For this review, use the dimensioned drawing (mm, ordinates from the lowest corner) and the shaded views. A direction names the side the tool comes from. Round coordinates to 2 decimals unless told otherwise and drop trailing zeros. Order: outer loops, then holes, each group sorted by start corner. A loop starts at its lowest first (then second) coordinate and runs counter-clockwise, first axis right, second up. Notation, with made-up numbers: (-31.5, 55) -> (-15.5, 55) arc R23 ccw to (-15.5, 86) -> close; hole circle Ø4 at (78, 72.25). An arc over 180 degrees is marked (long way). Answer in a Markdown table with one row per item.
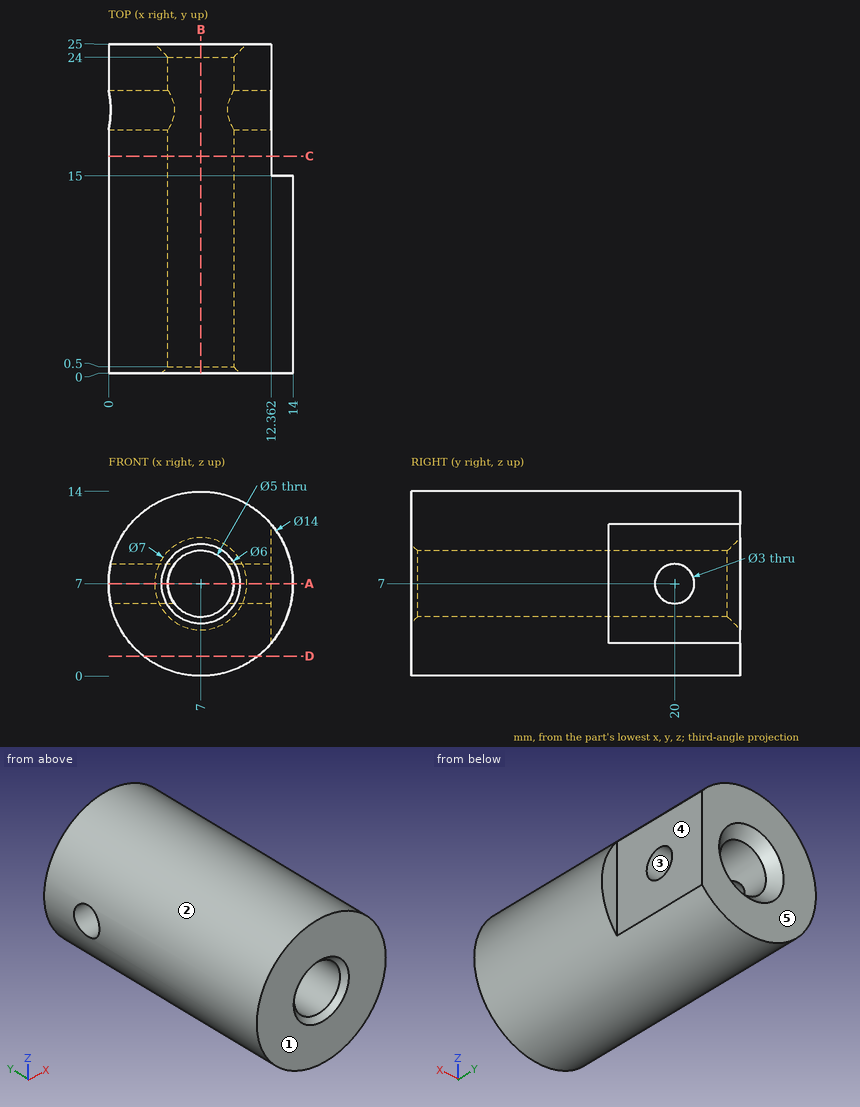
Q1. To check wall thickness, follow probe 1 along Z at (x, y) = (7, 17.75); probe 2 along Z at (x, y) = (5.5, 21.75); probe 3 along X at (y, z) = (15.5, 6.5). State the ranges of each line that lie inside material, in increasing order.
Answer key:
| item | result |
|---|---|
| probe 1 | z = 0 to 4.5, 9.5 to 14 |
| probe 2 | z = 0.16 to 5, 9 to 13.84 |
| probe 3 | x = 0.02 to 4.55, 9.45 to 12.36 |
Q2. Take a section at D-D, the plane z = 1.5. Write out the cut boundary in (x, y).
Answer key:
| item | result |
|---|---|
| outline | (2.67, 0) -> (11.33, 0) -> (11.33, 25) -> (2.67, 25) -> close |
Q3. Tool access review of the marked faces 4 and 5: name each direction out of +Z, -Z, +X, -X, +Y, -Y from which nothing blocks a thin tool from reaching the whole face with its end or side.
Answer key:
| item | result |
|---|---|
| face 4 | +Z, -Z, +X, +Y |
| face 5 | +Z, -Z, +X, -X, +Y |
Q4. The part is to be moulded in two halves that separate along Z. For the marked faces 1, 2 and 3, say which applies: +Z half, -Z half, draft (parallel to the pull), parting line (faces both ways), or undercut.
Answer key:
| item | result |
|---|---|
| face 1 | draft |
| face 2 | parting line |
| face 3 | undercut |
Q5. Take a section at C-C, the plane y = 16.5. Write out the cut boundary in (x, z), then the cut area to 3 significant figures.
Answer key:
| item | result |
|---|---|
| outline | (12.36, 2.5) -> (12.36, 11.5) arc R7 ccw (long way) to start; hole circle Ø5 at (7, 7) |
| area | 124 mm^2 |
Q6. Take a section at A-A, the plane z = 7. Write out the cut boundary in (x, y).
Answer key:
| item | result |
|---|---|
| outline | (0, 0) -> (4, 0) -> (4.5, 0.5) -> (4.5, 18.5) -> (0, 18.5) -> close; (0, 21.5) -> (4.5, 21.5) -> (4.5, 24) -> (3.5, 25) -> (0, 25) -> close; (9.5, 0.5) -> (10, 0) -> (14, 0) -> (14, 15) -> (12.36, 15) -> (12.36, 18.5) -> (9.5, 18.5) -> close; (9.5, 21.5) -> (12.36, 21.5) -> (12.36, 25) -> (10.5, 25) -> (9.5, 24) -> close |
Q7. Take a section at B-B, the plane x = 7. Write out the cut boundary in (y, z).
Answer key:
| item | result |
|---|---|
| outline | (0, 0) -> (25, 0) -> (25, 3.5) -> (24, 4.5) -> (0.5, 4.5) -> (0, 4) -> close; (0, 10) -> (0.5, 9.5) -> (24, 9.5) -> (25, 10.5) -> (25, 14) -> (0, 14) -> close |
Q8. Clearance check with flat-ended pins moving along their axes: pin 1 Ø4.5 at (y, z) = (18.5, 5) entering from +X; pin 2 Ø1 at (x, y) = (12.5, 7.5) entering from +Z; pin 3 Ø1 at (y, z) = (17.5, 4) entering from -X. State where each tip first meets the part, or that it passes through.
Answer key:
| item | result |
|---|---|
| pin 1 | stops at x = 12.36 |
| pin 2 | stops at z = 11.9 |
| pin 3 | stops at x = 0.46 |
